CAD build for the part. Positions are in the model's coordinates, mm. A direction names the side the tool comes from. Coordinates: 2 decimals unless noted, no trailing zeros. Order: outer loops, then holes, each group sorted by start corner. A loop starts at its lowest first (then second) coordinate and runs counter-clockwise, first axis right, second up. Notation, with made-up numbers: M 66.5,-31.5 L 116.5,-31.5 A24 cw 116.5,-3.5 Z; hole C 2,43.5 d5. An arc over 180 degrees is marked long. One line per item, written item: value.
Autodesk Inventor part; units mm, degrees
ref_plane "YZ Plane" through (0, 0, 0) normal (1, 0, 0) x (0, 1, 0)
ref_plane "XZ Plane" through (0, 0, 0) normal (0, 1, 0) x (-1, 0, 0)
ref_plane "XY Plane" through (0, 0, 0) normal (0, 0, 1) x (1, 0, 0)
sketch "Sketch1" plane through (0, 0, 0) normal (0, 0, 1) x (1, 0, 0)
  line L0 (-11.5, -148.5) -> (-11.5, -147.1375)
  line L1 (-21.5, -147.1375) -> (-21.5, -148.5)
  line L2 (-41, -148.5) -> (-41, 0.5)
  line L3 (-41, 0.5) -> (-21.5, 0.5)
  line L4 (-21.5, 0.5) -> (-21.5, -2.5)
  line L5 (-11.5, -2.5) -> (-11.5, 0.5)
  line L6 (-11.5, 0.5) -> (0, 0.5)
  line L7 (-11.5, -148.5) -> (-11.5, -147.1375)
  line L8 (-21.5, -147.1375) -> (-21.5, -148.5)
  line L9 (-41, -148.5) -> (-41, 0.5)
  line L10 (-41, 0.5) -> (-21.5, 0.5)
  line L11 (-21.5, 0.5) -> (-21.5, -2.5)
  line L12 (-11.5, -2.5) -> (-11.5, 0.5)
  line L13 (-11.5, 0.5) -> (0, 0.5)
  line L14 (-41, -150.3125) -> (-41, 0.5)
  line L15 (-11.5, -150.3125) -> (-11.5, -147.1375)
  line L16 (-11.5, -147.1375) -> (-21.5, -147.1375)
  line L17 (-21.5, -147.1375) -> (-21.5, -150.3125)
  line L18 (0, -150.3125) -> (-11.5, -150.3125)
  line L19 (-21.5, -150.3125) -> (-41, -150.3125)
  line L20 (-11.5, 0.5) -> (-11.5, -2.675)
  line L21 (-11.5, -2.675) -> (-21.5, -2.675)
  line L22 (-21.5, -2.675) -> (-21.5, 0.5)
  line L23 (0, 0.5) -> (-3.175, 0.5)
  line L24 (-3.175, -150.3125) -> (0, -150.3125)
  line L25 (-3.175, 0.5) -> (0, 0.5)
  line L26 (0, -9.66) -> (-2.9986, -9.66)
  line L27 (-2.9986, -9.66) -> (0, -9.66)
  line L28 (0, -19.82) -> (-2.9986, -19.82)
  line L29 (-2.9986, -19.82) -> (0, -19.82)
  line L30 (0, -39.7431) -> (-2.9986, -39.7431)
  line L31 (-2.9986, -39.7431) -> (0, -39.7431)
  line L32 (0, -49.9031) -> (-2.9986, -49.9031)
  line L33 (-2.9986, -49.9031) -> (0, -49.9031)
  line L34 (0, -69.8263) -> (-2.9986, -69.8263)
  line L35 (-2.9986, -69.8263) -> (0, -69.8263)
  line L36 (0, -79.9863) -> (-2.9986, -79.9863)
  line L37 (-2.9986, -79.9863) -> (0, -79.9863)
  line L38 (0, -99.9094) -> (-2.9986, -99.9094)
  line L39 (-2.9986, -99.9094) -> (0, -99.9094)
  line L40 (0, -110.0694) -> (-2.9986, -110.0694)
  line L41 (-2.9986, -110.0694) -> (0, -110.0694)
  line L42 (0, -129.9925) -> (-2.9986, -129.9925)
  line L43 (-2.9986, -129.9925) -> (0, -129.9925)
  line L44 (0, -140.1525) -> (-2.9986, -140.1525)
  line L45 (-2.9986, -140.1525) -> (0, -140.1525)
  line L46 (0, -150.3125) -> (-3.175, -150.3125)
  line L47 (-41, 0.5) -> (-21.5, 0.5)
  line L48 (-11.5, 0.5) -> (0, 0.5)
  line L49 (-2.9986, -9.66) -> (-2.9986, -19.82)
  line L50 (-2.9986, -39.7431) -> (-2.9986, -49.9031)
  line L51 (0, -49.9031) -> (0.1778, -49.9031)
  line L52 (0.1778, -49.9031) -> (0.1778, -69.8263)
  line L53 (0.1778, -69.8263) -> (0, -69.8263)
  line L54 (-2.9986, -69.8263) -> (-2.9986, -79.9863)
  line L55 (0, -79.9863) -> (0.1778, -79.9863)
  line L56 (0.1778, -79.9863) -> (0.1778, -99.9094)
  line L57 (0.1778, -99.9094) -> (0, -99.9094)
  line L58 (-2.9986, -99.9094) -> (-2.9986, -110.0694)
  line L59 (-2.9986, -129.9925) -> (-2.9986, -140.1525)
  line L60 (0.1778, -150.3125) -> (0, -150.3125)
  line L61 (0, -140.1525) -> (0.1778, -140.1525)
  line L62 (0, -129.9925) -> (0.1778, -129.9925)
  line L63 (0, -110.0694) -> (0.1778, -110.0694)
  line L64 (0.1778, -110.0694) -> (0.1778, -129.9925)
  line L65 (0.1778, -140.1525) -> (0.1778, -150.3125)
  line L66 (0, -39.7431) -> (0.1778, -39.7431)
  line L67 (0.1778, -39.7431) -> (0.1778, -19.82)
  line L68 (0.1778, -19.82) -> (0, -19.82)
  line L69 (0, -9.66) -> (0.1778, -9.66)
  line L70 (0.1778, -9.66) -> (0.1778, 0.5)
  line L71 (0.1778, 0.5) -> (0, 0.5)
  point P0 (0, 0)
  dimension "d2" = 3.175
  dimension "d4" = 10.16
  dimension "d5" = 10.16
  dimension "d6" = 19.9231
  dimension "d7" = 10.16
  dimension "d8" = 19.9231
  dimension "d9" = 10.16
  dimension "d10" = 19.9231
  dimension "d13" = 10.16
extrude "Extrusion2" add sketch "Sketch1" along normal blind 3.175
properties part number "1-8inch_Bottom2_1-Part"
Q1. Drill centre lines: line 1 along X through (y, z) = (-135, 2.7); line 2 along Y through (x, z) = (-14, 1.95) (1 decimal). Where is each one in solid material? Low to high.
Recorded:
line 1: x = -41 to -3
line 2: y = -147.1 to -2.7
Q2. Pin check, flat tips, straight feed: pin 1 Ø1 at (x, z) = (-19, 1) entering from -Y; pin 2 Ø1.6 at (y, z) = (-106.5, 2) entering from +X; pin 3 Ø1 at (x, z) = (-16, 2.5) entering from +Y (3 decimals). Stop position of each tip, or through.
Recorded:
pin 1: stops at y = -147.14
pin 2: stops at x = -3
pin 3: stops at y = -2.675
Q3. Mould opens along X. For faces 1 (the face through (-21.5, -1, 2)), 2 (the face through (-31, 0.5, 2)), 3 (the face through (-2.999, -75, 2)) say: released by +X, released by -X, zero draft, split by the parting line, or undercut.
Recorded:
face 1: undercut
face 2: zero draft
face 3: released by +X
Q4. Slice it at C-C (y = -44). List the corners of the cut face in (x, z) (3 decimals).
Recorded:
outline: M -41,0 L -2.999,0 L -2.999,3.175 L -41,3.175 Z
Q5. Slice it at B-B (x = -20). List the corners of the cut face in (y, z) (1 decimal).
Recorded:
outline: M -147.1,0 L -2.7,0 L -2.7,3.2 L -147.1,3.2 Z
Q6. Which spindle directions (+Z, -Z, +X, -X, +Y, -Y) get a long thin tool onto all of the face, cutting with end or side? Do faces 4 (the face through (-2.999, -105, 2)), 5 (the face through (-21, -74, 3.175)), 6 (the face through (-11.5, -149, 2)), 7 (the face through (-16, -2.675, 2)). Say none if no direction does.
Recorded:
face 4: +Z, -Z, +X
face 5: +Z, +X, -X, +Y, -Y
face 6: +Z, -Z, -Y
face 7: +Z, -Z, +Y
